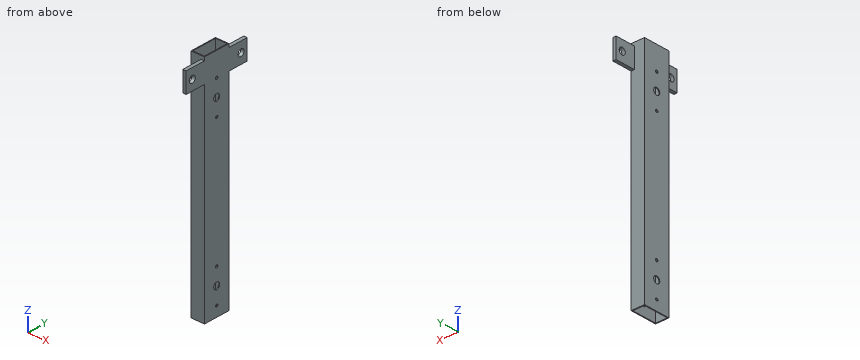
Autodesk Inventor part; units mm, degrees
ref_plane "XY Plane" through (0, 0, 0) normal (0, 0, 1) x (1, 0, 0)
sketch "Sketch1" plane through (0, 0, 0) normal (0, 0, 1) x (1, 0, 0)
  line L0 (-12.7, -25.4) -> (12.7, -25.4)
  line L1 (12.7, -25.4) -> (12.7, 25.4)
  line L2 (12.7, 25.4) -> (-12.7, 25.4)
  line L3 (-12.7, 25.4) -> (-12.7, -25.4)
  line L4 (-12.7, -25.4) -> (12.7, 25.4) construction
  line L5 (12.7, -25.4) -> (-12.7, 25.4) construction
  line L6 (-11.049, -23.749) -> (11.049, -23.749)
  line L7 (11.049, -23.749) -> (11.049, 23.749)
  line L8 (11.049, 23.749) -> (-11.049, 23.749)
  line L9 (-11.049, 23.749) -> (-11.049, -23.749)
  line L10 (-11.049, -23.749) -> (11.049, 23.749) construction
  line L11 (11.049, -23.749) -> (-11.049, 23.749) construction
  point P0 (0, 0)
  dimension "d0" = 25.4
  dimension "d1" = 50.8
  dimension "d4" = 22.098
  dimension "d5" = 47.498
extrude "Extrusion2" add sketch "Sketch1" along normal mid plane 431.8
sketch "Sketch2" plane through (12.7, -25.4, 215.9) normal (1, 0, 0) x (0, 0, -1)
  line L0 (431.8, 50.8) -> (0, 50.8)
  line L1 (0, 0) -> (0, 50.8)
  line L2 (431.8, 0) -> (0, 0)
  line L3 (431.8, 50.8) -> (431.8, 0)
  point P0 (215.9, 25.4)
  point P1 (76.2, 25.4)
  dimension "d8" = 76.2
  dimension "d9" = 25.4
hole "Hole1" at (12.7, 0, 139.7) direction (-1, 0, 0) diameter 12.7 end through all
ref_plane "Work Plane1" through (-12.7, -25.4, 215.9) normal (-1, 0, 0) x (0, 0, 1)
ref_plane "Work Plane2" through (12.7, -25.4, 215.9) normal (-1, 0, 0) x (0, 0, 1)
sketch "Sketch4" plane through (-12.7, -25.4, 215.9) normal (-1, 0, 0) x (0, 0, 1)
  circle A0 centre (-76.2, 25.4) radius 6.35
  line L0 (0, 0) -> (-431.8, 0)
  line L1 (0, 50.8) -> (0, 0)
  line L2 (-431.8, 50.8) -> (0, 50.8)
  line L3 (-431.8, 0) -> (-431.8, 50.8)
  point P0 (-215.9, 25.4)
  point P1 (-381, 25.4)
  dimension "d29" = 50.8
  dimension "d30" = 25.4
hole "Hole3" at (-12.7, 0, -165.1) direction (1, 0, 0) diameter 12.7 end through all
sketch "Sketch5" plane through (-12.7, -25.4, 215.9) normal (-1, 0, 0) x (0, 0, 1)
  circle A0 centre (-381, 25.4) radius 6.35
  circle A1 centre (-76.2, 25.4) radius 6.35
  line L0 (0, 0) -> (-431.8, 0)
  line L1 (0, 50.8) -> (0, 0)
  line L2 (-431.8, 50.8) -> (0, 50.8)
  line L3 (-431.8, 0) -> (-431.8, 50.8)
  point P0 (-215.9, 25.4)
  point P1 (-412.75, 25.4)
  point P2 (-349.25, 25.4)
  dimension "d38" = 31.75
  dimension "d39" = 63.5
hole "Hole4" at (-12.7, 0, -133.35) at (-12.7, 0, -196.85) direction (1, 0, 0) diameter 5.08 end through all
ref_plane "Work Plane3" through (-12.7, 25.4, 215.9) normal (0, 1, 0) x (1, 0, 0)
sketch "Sketch6" plane through (12.7, -25.4, 215.9) normal (1, 0, 0) x (0, 0, -1)
  circle A0 centre (412.75, 25.4) radius 2.54
  circle A1 centre (349.25, 25.4) radius 2.54
  circle A2 centre (381, 25.4) radius 6.35
  circle A3 centre (76.2, 25.4) radius 6.35
  line L0 (431.8, 50.8) -> (0, 50.8)
  line L1 (0, 0) -> (0, 50.8)
  line L2 (431.8, 0) -> (0, 0)
  line L3 (431.8, 50.8) -> (431.8, 0)
  circle A4 centre (25.4, 76.2) radius 6.35
  line L4 (6.35, 50.8) -> (44.45, 50.8)
  line L5 (44.45, 50.8) -> (44.45, 88.9)
  line L6 (44.45, 88.9) -> (6.35, 88.9)
  line L7 (6.35, 88.9) -> (6.35, 50.8)
  point P0 (215.9, 25.4)
  dimension "d48" = 12.7
  dimension "d49" = 25.4
  dimension "d50" = 25.4
  dimension "d51" = 38.1
  dimension "d52" = 38.1
  dimension "d53" = 19.05
extrude "Extrusion3" add sketch "Sketch6" against normal blind 6.35 contours L0 L7 L6 L5
mirror "Mirror2" about plane through (0, 0, 0) normal (0, 1, 0) of "Extrusion3"
pattern_linear "Rectangular Pattern1" count 2 spacing 304.8 along (0, 0, 1) of "Hole4"
properties part number "Steel 4130 1x2in. Tubing, t=.065in.,L=22in." material "Steel"
Read the model definition and answer for the solid it produces. Units are mm, in the model's axes. Coordinates: 2 decimals unless noted, no trailing zeros. Loops run counter-clockwise (first coordinate to the right, second up) from the corner with the lowest first, then second, coordinate; pieces in that order, holes last. Notation, with made-up numbers: (10.25, 44) -> (55.25, 44) arc R30 ccw to (55.25, 82) -> close; hole circle Ø6 at (5, -8). An arc over 180 degrees is marked (long way). Write item = value, one per line. Start each with the question number.
1) The part is cut by section D-D, the plane z = -165.1. Determine the outline of the cut face in (x, y).
2) Find the intervals of material crossed by L1, parallel to Y at x = 9.5, z = 190.5; L2, parallel to Y at x = -6, z = -163; L3, parallel to Y at x = 11.25, z = 190.5, in increasing order. Write a range as from..to.
3) The part is cut by section A-A, the plane z = 190.5. Determine the outline of the cut face in (x, y), plus the area to 3 significant figures.
4) The part is cut by section C-C, the plane x = -2.25. Determine the outline of the cut face in (y, z), plus the area to 3 significant figures.
5) The part is cut by section B-B, the plane y = -50.8. Determine the outline of the cut face in (x, z).
6) Given P1, Ø5, axis at x = 9.5, z = -92, coming from the +Y side; P2, Ø11.5, axis at y = 0, z = -165.1, coming from the +X side; P3, Ø1.5, axis at x = -8, z = 16.5, coming from the -Y side; P4, Ø5, axis at x = 8.5, y = 50.5, coming from the -Z side, each flat-ended and moving along its own axis, determine where each tip first touches the part or whether it passes through.
Result:
q1.outline = (-12.7, -25.4) -> (12.7, -25.4) -> (12.7, -6.35) -> (11.05, -6.35) -> (11.05, -23.75) -> (-11.05, -23.75) -> (-11.05, -6.35) -> (-12.7, -6.35) -> close; (-12.7, 6.35) -> (-11.05, 6.35) -> (-11.05, 23.75) -> (11.05, 23.75) -> (11.05, 6.35) -> (12.7, 6.35) -> (12.7, 25.4) -> (-12.7, 25.4) -> close
q2.L1 = -63.5..-57.15, -44.45..-23.75, 23.75..44.45, 57.15..63.5
q2.L2 = -25.4..-23.75, 23.75..25.4
q2.L3 = -63.5..-57.15, -44.45..44.45, 57.15..63.5
q3.outline = (-12.7, -25.4) -> (6.35, -25.4) -> (6.35, -44.45) -> (12.7, -44.45) -> (12.7, 44.45) -> (6.35, 44.45) -> (6.35, 25.4) -> (-12.7, 25.4) -> close; (6.35, -63.5) -> (12.7, -63.5) -> (12.7, -57.15) -> (6.35, -57.15) -> close; (6.35, 57.15) -> (12.7, 57.15) -> (12.7, 63.5) -> (6.35, 63.5) -> close; hole (-11.05, -23.75) -> (11.05, -23.75) -> (11.05, 23.75) -> (-11.05, 23.75) -> close
q3.area = 563 mm²
q4.outline = (-25.4, -215.9) -> (-23.75, -215.9) -> (-23.75, 215.9) -> (-25.4, 215.9) -> close; (23.75, -215.9) -> (25.4, -215.9) -> (25.4, 215.9) -> (23.75, 215.9) -> close
q4.area = 1,430 mm²
q5.outline = (6.35, 171.45) -> (12.7, 171.45) -> (12.7, 184.15) -> (6.35, 184.15) -> close; (6.35, 196.85) -> (12.7, 196.85) -> (12.7, 209.55) -> (6.35, 209.55) -> close
q6.P1 = 25.4
q6.P2 = through
q6.P3 = -25.4
q6.P4 = 171.45
